Read the model definition and answer for the solid it produces. Units are mm, in the model's axes. A direction names the side the tool comes from. Give positions to 0.01 mm unless a question says otherwise; leave off trailing zeros. Write each loop counter-clockwise with the first axis right and the second up, starting at its lowest first coordinate (ties: lowest second). Pieces come first, ordered by that corner, then holes. Notation, with made-up numbers: M -32.5,57 L 2.5,57 A23 ccw 2.5,90 Z; hole C 73,84 d7. An arc over 180 degrees is marked long. Use a Markdown table: item, result. Add a question column.
Item 1: The mould has two halves that part along Y. Classify faces 4 (the flat face through (40, -70, 3)), 5 (the flat face through (94, -27, 3)), 6 (the flat face through (-7.5, -44, 3)): pulls with the +Y half, pulls with the -Y half, needs draft (parallel to the pull), parting line crosses it, or undercut.
Item 2: A cutting plane is placed at A-A on y = -47.5. Determine the outline of the cut face in (x, z).
Item 3: A cutting plane is placed at C-C on x = -86.5. Determine the outline of the cut face in (y, z), then the cut area to 3 significant figures.
Item 4: Consider probe 1 along Y at (x, z) = (-21.5, 3.7); probe 2 along Y at (x, z) = (3, 4.45); probe 3 along X at (y, z) = (-5.5, 1.6). Determine where each line is inside the solid, lowest interval first. Write a range as [from, to].
Item 5: For faces 1 (the flat face through (-64, -51, 3)), 2 (the flat face through (-79, 28, 3)), 3 (the flat face through (64, -51, 3)), determine the directions among +Z, -Z, +X, -X, +Y, -Y from which every point of the face is accessible in a straight line to the end or side of a thin tool.
Item 6: A cutting plane is placed at D-D on y = 61. Determine the outline of the cut face in (x, z), then the cut area to 3 significant figures.
Item 7: A cutting plane is placed at B-B on z = 3.35. Count the separate pieces of the cut face and the enclosed holes in it, then the cut area to 3 significant figures.
Item 8: Given P1, Ø1, axis at x = 17, z = 3.5, coming from the -Y side; P2, Ø1.8, axis at y = 43, z = 4, coming from the -X side; P3, Ø1.8, axis at y = -66, z = 4.5, coming from the +X side; P4, Ø10, axis at x = -59.5, y = 31, coming from the -Z side, each flat-ended and moving along its own axis, determine where each tip first touches the part or whether it passes through.
from build123d import *

# Parameters (mm, degrees)
BOSS_EXTRU_3_DEPTH      = 6
ESQUISSE2_W             = 3
ESQUISSE2_H             = 10
ENL_V_MAT_EXTRU_1_DEPTH = 10
ESQUISSE3_W             = 30
ESQUISSE3_H             = 26
ENL_V_MAT_EXTRU_2_DEPTH = 6
ESQUISSE4_W             = 15
ESQUISSE4_H             = 20
ENL_V_MAT_EXTRU_3_DEPTH = 6
ESQUISSE5_W             = 10
ESQUISSE5_H             = 56
ENL_V_MAT_EXTRU_4_DEPTH = 6
ESQUISSE6_R             = 1
ENL_V_MAT_EXTRU_5_DEPTH = 123.21292894
ESQUISSE7_W             = 16
ESQUISSE7_H             = 6
ENL_V_MAT_EXTRU_6_DEPTH = 1


with BuildPart() as part:
    # Esquisse1 → Boss.-Extru.3 (new body)
    with BuildSketch(Plane.XY):
        Polygon((-94, 64), (-94, 15), (-100, 15), (-100, -15), (-94, -15), (-94, -64), (-60, -64), (-60, -70), (-20, -70), (-20, -64), (20, -64), (20, -70), (60, -70), (60, -64), (94, -64), (94, -15), (100, -15), (100, 15), (94, 15), (94, 64), (54, 64), (54, 70), (24, 70), (24, 64), (-24, 64), (-24, 70), (-54, 70), (-54, 64), align=None)
    extrude(amount=BOSS_EXTRU_3_DEPTH)

    # Esquisse2 → Enlèv. mat.-Extru.1 (cut)
    with BuildSketch(Plane.XY.offset(6)):
        with Locations((-65.5, -23)):
            Rectangle(ESQUISSE2_W, ESQUISSE2_H)
        with Locations((-65.5, 23)):
            Rectangle(ESQUISSE2_W, ESQUISSE2_H)
        with Locations((-14.5, -23)):
            Rectangle(ESQUISSE2_W, ESQUISSE2_H)
        with Locations((-14.5, 23)):
            Rectangle(ESQUISSE2_W, ESQUISSE2_H)
        with Locations((65.5, -23)):
            Rectangle(ESQUISSE2_W, ESQUISSE2_H)
        with Locations((14.5, 23)):
            Rectangle(ESQUISSE2_W, ESQUISSE2_H)
        with Locations((14.5, -23)):
            Rectangle(ESQUISSE2_W, ESQUISSE2_H)
        with Locations((65.5, 23)):
            Rectangle(ESQUISSE2_W, ESQUISSE2_H)
    extrude(amount=-ENL_V_MAT_EXTRU_1_DEPTH, mode=Mode.SUBTRACT)

    # Esquisse3 → Enlèv. mat.-Extru.2 (cut)
    with BuildSketch(Plane.XY.offset(6)):
        with Locations((79, -51)):
            Rectangle(ESQUISSE3_W, ESQUISSE3_H)
        with Locations((-79, -51)):
            Rectangle(ESQUISSE3_W, ESQUISSE3_H)
        with Locations((-79, 51)):
            Rectangle(ESQUISSE3_W, ESQUISSE3_H)
        with Locations((79, 51)):
            Rectangle(ESQUISSE3_W, ESQUISSE3_H)
    extrude(amount=-ENL_V_MAT_EXTRU_2_DEPTH, mode=Mode.SUBTRACT)

    # Esquisse4 → Enlèv. mat.-Extru.3 (cut)
    with BuildSketch(Plane(origin=(0, 0, 0), x_dir=(-1, 0, 0), z_dir=(0, 0, -1))):
        with Locations((0, -44)):
            Rectangle(ESQUISSE4_W, ESQUISSE4_H)
        with Locations((0, 44)):
            Rectangle(ESQUISSE4_W, ESQUISSE4_H)
    extrude(amount=-ENL_V_MAT_EXTRU_3_DEPTH, mode=Mode.SUBTRACT)

    # Esquisse5 → Enlèv. mat.-Extru.4 (cut)
    with BuildSketch(Plane(origin=(0, 0, 0), x_dir=(-1, 0, 0), z_dir=(0, 0, -1))):
        with Locations((-79, 0)):
            Rectangle(ESQUISSE5_W, ESQUISSE5_H)
        with Locations((79, 0)):
            Rectangle(ESQUISSE5_W, ESQUISSE5_H)
    extrude(amount=-ENL_V_MAT_EXTRU_4_DEPTH, mode=Mode.SUBTRACT)

    # Esquisse6 → Enlèv. mat.-Extru.5 (cut, through all)
    with BuildSketch(Plane(origin=(0, 0, 0), x_dir=(-1, 0, 0), z_dir=(0, 0, -1))):
        with Locations((21.5, -35)):
            Circle(ESQUISSE6_R)
        with Locations((21.5, 5)):
            Circle(ESQUISSE6_R)
        with Locations(Location((-21.5, 5, 0), (0, 0, 180))):
            Circle(ESQUISSE6_R)
        with Locations(Location((-21.5, -35, 0), (0, 0, 180))):
            Circle(ESQUISSE6_R)
    extrude(amount=-ENL_V_MAT_EXTRU_5_DEPTH, mode=Mode.SUBTRACT)

    # Esquisse7 → Enlèv. mat.-Extru.6 (cut)
    with BuildSketch(Plane(origin=(0, 0, 0), x_dir=(-1, 0, 0), z_dir=(0, 0, -1))):
        with Locations((21.5, -35)):
            Rectangle(ESQUISSE7_W, ESQUISSE7_H)
        with Locations((21.5, 5)):
            Rectangle(ESQUISSE7_W, ESQUISSE7_H)
        with Locations((-21.5, 5)):
            Rectangle(ESQUISSE7_W, ESQUISSE7_H)
        with Locations((-21.5, -35)):
            Rectangle(ESQUISSE7_W, ESQUISSE7_H)
    extrude(amount=-ENL_V_MAT_EXTRU_6_DEPTH, mode=Mode.SUBTRACT)


solid = part.part
Filled in:
| question | item | result |
|---|---|---|
| 1 | face 4 | pulls with the -Y half |
| 1 | face 5 | needs draft |
| 1 | face 6 | undercut |
| 2 | outline | M -64,0 L -7.5,0 L -7.5,6 L -64,6 Z; M 7.5,0 L 64,0 L 64,6 L 7.5,6 Z |
| 3 | outline | M -38,0 L 38,0 L 38,6 L -38,6 Z |
| 3 | area | 456 mm² |
| 4 | probe 1 | [-70, -36], [-34, 4], [6, 64] |
| 4 | probe 2 | [-64, -54], [-34, 34], [54, 64] |
| 4 | probe 3 | [-100, -84], [-74, 74], [84, 100] |
| 5 | face 1 | +Z, -Z, -X, -Y |
| 5 | face 2 | +Z, -Z |
| 5 | face 3 | +Z, -Z, +X, -Y |
| 6 | outline | M -64,0 L 64,0 L 64,6 L -64,6 Z |
| 6 | area | 768 mm² |
| 7 | separate pieces | 1 |
| 7 | enclosed holes | 16 |
| 7 | area | 20,200 mm² |
| 8 | P1 | y = -64 |
| 8 | P2 | x = -64 |
| 8 | P3 | x = 60 |
| 8 | P4 | z = 0 |
